```python
from build123d import *

# Parameters (mm, degrees)
SKETCH1_R           = 8.255
BOSS_EXTRUDE1_DEPTH = 2.3368
SKETCH2_R           = 2.38125
BOSS_EXTRUDE2_DEPTH = 17.78


with BuildPart() as part:
    # Sketch1 → Boss-Extrude1 (new body)
    with BuildSketch(Plane.XY):
        Circle(SKETCH1_R)
    extrude(amount=BOSS_EXTRUDE1_DEPTH)

    # Sketch2 → Boss-Extrude2 (add)
    with BuildSketch(Plane.XY):
        Circle(SKETCH2_R)
    extrude(amount=-BOSS_EXTRUDE2_DEPTH)

    # Sketch3 → Cut-Revolve1 (revolve, cut)
    with BuildSketch(Plane(origin=(0, 0, 0), x_dir=(1, 0, 0), z_dir=(0, 1, 0))):
        with BuildLine():
            ThreePointArc((1.4478, -2.3368), (4.989096566, -1.838155581), (8.255, -0.381))
            Line((8.255, -0.381), (8.255, -2.3368))
            Line((8.255, -2.3368), (1.4478, -2.3368))
        make_face()
    revolve(axis=Axis((0, 0, 2.3368), (0, 0, -1)), mode=Mode.SUBTRACT)


solid = part.part
```
Work out the finished part from the listing and answer in its coordinate system (mm). A direction names the side the tool comes from. Round coordinates to 2 decimals unless told otherwise and drop trailing zeros. Loops run counter-clockwise (first coordinate to the right, second up) from the corner with the lowest first, then second, coordinate; pieces in that order, holes last. Notation, with made-up numbers: (47.25, 75) -> (54.25, 75) arc R9 cw to (54.25, 88) -> close; hole circle Ø2 at (46.25, -32). An arc over 180 degrees is marked (long way). Write each question's results on one line, items separated by ' | '. Start each with the question number.
1. Given pin 1 Ø8 at (x, y) = (3, 5.5) entering from +Z; pin 2 Ø3 at (x, z) = (-3, -3) entering from +Y; pin 3 Ø6 at (y, z) = (-2.5, -4.5) entering from +X, each flat-ended and moving along its own axis, determine where each tip first touches the part or whether it passes through.
2. Find the intervals of material crossed by probe 1 along Y at (x, z) = (-1.25, -4.5); probe 2 along Z at (x, y) = (-5.25, -5.5); probe 3 along X at (y, z) = (0.5, -3.5), in increasing order. Write a range as from..to.
3. A tool of negligible diameter and unlimited length cuts with its end or side. For faces 1 (the face through (2, -2, 0)), 2 (the face through (0, 0, -17.78)), from which of +Z, -Z, +X, -X, +Y, -Y can it reach the whole face along a straight path? Write none if from no direction.
4. Section A-A (z = -16.5) is taken. Determine the outline of the cut face in (x, y), plus the area to 3 significant figures.
5. For a pull along X with two mould halves and no side action, classify faces 3 (the face through (7.874, 2.48, 0.188)), 4 (the face through (0, 0, 2.337)) as +X half, -X half, draft (parallel to the pull), parting line (faces both ways), or undercut.
Evaluation:
1) pin 1: stops at z = 2.31 | pin 2: stops at y = 1.85 | pin 3: stops at x = 2.38
2) probe 1: y = -2.03..2.03 | probe 2: z = 0..0.76 | probe 3: x = -2.33..2.33
3) face 1: -Z | face 2: -Z, +X, -X, +Y, -Y
4) outline: circle Ø4.76 at (0, 0) | area: 17.8 mm2
5) face 3: parting line | face 4: draft
